```python
from build123d import *

# Parameters (mm, degrees)
F0_W      = 35
F0_H      = 25
F0_R      = 2.5
F1_DEPTH  = 40
F2_W      = 35
F2_H      = 25
F3_DEPTH  = 23
F4_W      = 35
F4_H      = 5
F5_DEPTH  = 10
F6_W      = 35
F6_H      = 7
F7_DEPTH  = 10
F8_W      = 25
F8_H      = 7
F9_DEPTH  = 7
F10_W     = 9.1652874053
F10_H     = 3
F11_DEPTH = 8
F14_D     = 4
F14_DEPTH = 3.001


with BuildPart() as f1:
    # F0 (on Top) → F1 (new body)
    with BuildSketch(Plane.XY):
        with Locations((-0.2066092566, 0)):
            Rectangle(F0_W, F0_H)
        Circle(F0_R, mode=Mode.SUBTRACT)
    extrude(amount=F1_DEPTH)

    # F2 (on face) → F3 (join)
    with BuildSketch(Plane.XY.offset(40)):
        with Locations((-0.2066092566, 0)):
            Rectangle(F2_W, F2_H)
    extrude(amount=F3_DEPTH)

    # F4 (on face) → F5 (join)
    with BuildSketch(Plane.XY.offset(63)):
        with Locations((-0.2066092566, 10)):
            Rectangle(F4_W, F4_H)
    extrude(amount=F5_DEPTH)

    # F6 (on face) → F7 (join)
    with BuildSketch(Plane.XY.offset(63)):
        with Locations((-0.2066092566, -1)):
            Rectangle(F6_W, F6_H)
    extrude(amount=F7_DEPTH)

    # F8 (on face) → F9 (cut)
    with BuildSketch(Plane.XZ.offset(4.5)):
        with Locations((-0.2066092566, 66.5)):
            Rectangle(F8_W, F8_H)
    extrude(amount=-F9_DEPTH, mode=Mode.SUBTRACT)

    # F10 (on face) → F11 (join)
    with BuildSketch(Plane.XY.offset(63)):
        with Locations((-0.1239655539, -11)):
            Rectangle(F10_W, F10_H)
    extrude(amount=F11_DEPTH)

    # F14 (through all, one way)
    with BuildSketch(Plane(origin=(0, -9.5, 0), x_dir=(-1, 0, 0), z_dir=(0, 1, 0))):
        with Locations((0, 66.9974908233)):
            Circle(F14_D / 2)
    extrude(amount=-F14_DEPTH, mode=Mode.SUBTRACT)


solid = f1.part
```
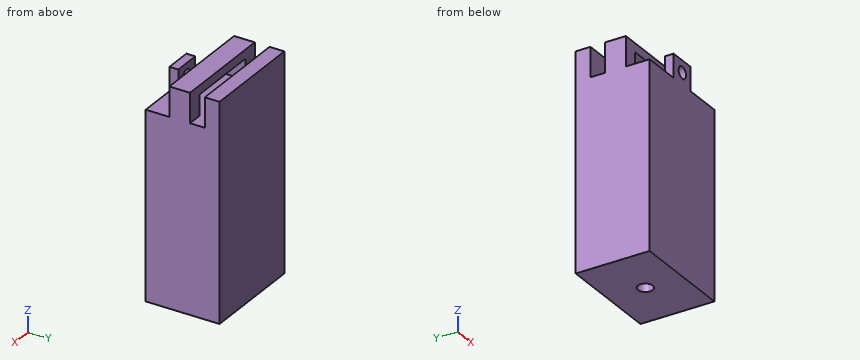
Can you work these out from the model? Positions are in its coordinate system, mm. Coordinates: 2 decimals unless noted, no trailing zeros. Loops run counter-clockwise (first coordinate to the right, second up) from the corner with the lowest first, then second, coordinate; pieces in that order, holes last. Notation, with made-up numbers: (-10.75, 29) -> (1.25, 29) arc R17 ccw to (1.25, 36) -> close; hole circle Ø5 at (19, -29). An arc over 180 degrees is marked (long way). Put each result on its own line as item: value. Start each with the question number.
Q1. I want a section at C-C (y = 0). Write out the boundary of the cut face in (x, z).
Q2. I'm going to push flat-ended pins straight in: P1, Ø0.9, axis at y = -10.5, z = 67, coming from the -X side; P2, Ø1, axis at x = -13.5, y = -7, coming from the +Z side; P3, Ø1.5, axis at x = -0.5, y = 0.5, coming from the -Z side. Where does each tip first touch, or does it pass through?
Q3. I want a section at B-B (x = 0). Write out the boundary of the cut face in (y, z), plus the area to 3 significant figures.
Q4. If I drill on line 1 (Z direction, x = 4.5, y = -0.25); line 2 (Y direction, x = 1, z = 69.5); line 3 (Z direction, x = 0, y = -10.65), over which ranges is the centre line in solid material (lowest first)? Write a range as [from, to].
Q5. I want a section at A-A (x = -11.5). Write out the boundary of the cut face in (y, z).
Q6. I want a section at D-D (z = 21.5). Write out the boundary of the cut face in (x, y).
Taken from the geometry:
1. outline: (-17.71, 0) -> (-2.5, 0) -> (-2.5, 40) -> (2.5, 40) -> (2.5, 0) -> (17.29, 0) -> (17.29, 73) -> (-17.71, 73) -> close; hole (-12.71, 63) -> (12.29, 63) -> (12.29, 70) -> (-12.71, 70) -> close
2. P1: stops at x = -4.71
2. P2: stops at z = 63
2. P3: stops at z = 40
3. outline: (-12.5, 0) -> (-2.5, 0) -> (-2.5, 40) -> (2.5, 40) -> (2.5, 0) -> (12.5, 0) -> (12.5, 73) -> (7.5, 73) -> (7.5, 63) -> (-9.5, 63) -> (-9.5, 65) -> (-12.5, 65) -> close; (-12.5, 69) -> (-9.5, 69) -> (-9.5, 71) -> (-12.5, 71) -> close; (-4.5, 70) -> (2.5, 70) -> (2.5, 73) -> (-4.5, 73) -> close
3. area: 1,460 mm2
4. line 1: z = [0, 63], [70, 73]
4. line 2: y = [-12.5, -9.5], [7.5, 12.5]
4. line 3: z = [0, 65], [69, 71]
5. outline: (-12.5, 0) -> (12.5, 0) -> (12.5, 73) -> (7.5, 73) -> (7.5, 63) -> (-12.5, 63) -> close; (-4.5, 70) -> (2.5, 70) -> (2.5, 73) -> (-4.5, 73) -> close
6. outline: (-17.71, -12.5) -> (17.29, -12.5) -> (17.29, 12.5) -> (-17.71, 12.5) -> close; hole circle Ø5 at (0, 0)
